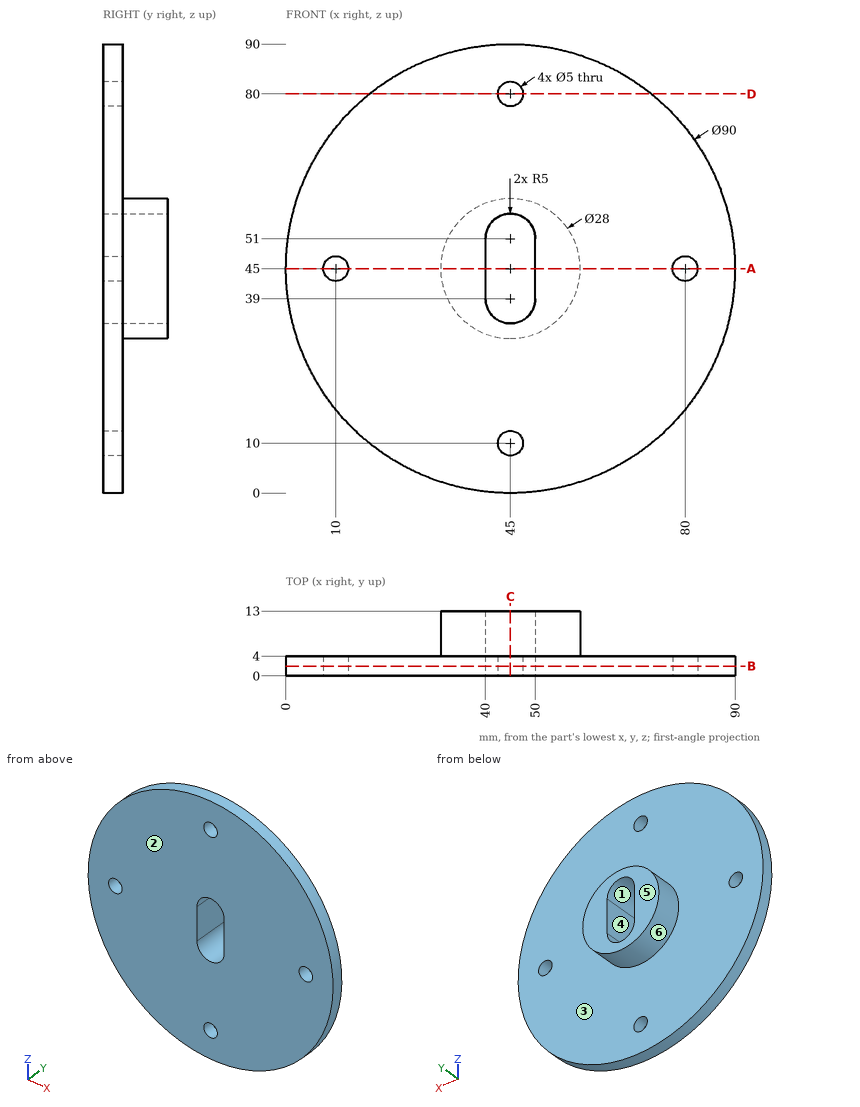
Verification items for this drawing (mm, ordinates from the low corner). A direction names the side the tool comes from. Coordinates: 2 decimals unless noted, no trailing zeros. Write each loop counter-clockwise with the first axis right and the second up, starting at its lowest first coordinate (ties: lowest second). Pieces come first, ordered by that corner, then holes. Notation, with made-up numbers: M -13.75,86.5 L 45.25,86.5 A19 ccw 45.25,98.5 Z; hole C -6.5,69 d1. An arc over 180 degrees is marked long. Answer as a JSON object with one key per item and string values.
1. Scan lines: L1, parallel to X at y = 2.95, z = 45; L2, parallel to Y at x = 62, z = 69; L3, parallel to Z at x = 10, y = 1.25. Record each from-to range of solid material in increasing order.
Answers below:
{"L1": "x = 0 to 7.5, 12.5 to 40, 50 to 77.5, 82.5 to 90", "L2": "y = 0 to 4", "L3": "z = 16.72 to 42.5, 47.5 to 73.28"}
2. Go/stop test with flat-tipped pins: pin 1 Ø4.5 at (x, z) = (45, 10) entering from +Y (3 decimals); pin 2 Ø2 at (y, z) = (3, 52) entering from -X; pin 3 Ø3 at (x, y) = (18.5, 2) entering from +Z; pin 4 Ø1 at (x, z) = (73, 50) entering from +Y. Record where each tip stops, or that it passes through.
Answers below:
{"pin 1": "passes through", "pin 2": "stops at x = 0.4", "pin 3": "stops at z = 82.42", "pin 4": "stops at y = 4"}
3. Section check C-C, the plane x = 45. Enter the section's corners in (y, z).
Answers below:
{"outline": "M 0,0 L 4,0 L 4,7.5 L 0,7.5 Z; M 0,12.5 L 4,12.5 L 4,31 L 13,31 L 13,34 L 0,34 Z; M 0,56 L 13,56 L 13,59 L 4,59 L 4,77.5 L 0,77.5 Z; M 0,82.5 L 4,82.5 L 4,90 L 0,90 Z"}
4. Section check A-A, the plane z = 45. Enter the section's corners in (x, y).
Answers below:
{"outline": "M 0,0 L 7.5,0 L 7.5,4 L 0,4 Z; M 12.5,0 L 40,0 L 40,13 L 31,13 L 31,4 L 12.5,4 Z; M 50,0 L 77.5,0 L 77.5,4 L 59,4 L 59,13 L 50,13 Z; M 82.5,0 L 90,0 L 90,4 L 82.5,4 Z"}
5. Section check D-D, the plane z = 80. Enter the section's corners in (x, y), plus the area to 3 significant figures.
Answers below:
{"outline": "M 16.72,0 L 42.5,0 L 42.5,4 L 16.72,4 Z; M 47.5,0 L 73.28,0 L 73.28,4 L 47.5,4 Z", "area": "206 mm²"}
6. Tool access check on the marked faces 1, 2 and 3. Record the directions out of +Z, -Z, +X, -X, +Y, -Y that give a thin tool (end or side, any length) a straight path to the whole face; none if there is none.
Answers below:
{"face 1": "+Y, -Y", "face 2": "+Z, -Z, +X, -X, -Y", "face 3": "+Y"}
7. Section check B-B, the plane y = 2. Enter the section's corners in (x, z), plus the area to 3 significant figures.
Answers below:
{"outline": "C 45,45 d90; hole C 10,45 d5; hole M 40,39 A5 ccw 50,39 L 50,51 A5 ccw 40,51 Z; hole C 45,10 d5; hole C 45,80 d5; hole C 80,45 d5", "area": "6,080 mm²"}
8. Draft check along X on the marked faces 4, 5 and 6. Enter one of: released by +X, released by -X, zero draft, split by the parting line, or undercut.
Answers below:
{"face 4": "undercut", "face 5": "zero draft", "face 6": "split by the parting line"}
